from build123d import *

# Parameters (mm, degrees)
EXTRUDE_1_DEPTH      = 50
SKETCH_1_4_R         = 5.1
CUT_EXTRUDE_1_DEPTH  = 45
CUT_EXTRUDE_2_DEPTH  = 5
SKETCH_1_6_R         = 5.1
CUT_EXTRUDE_3_DEPTH  = 5
SKETCH_1_7_R         = 2.6
CUT_EXTRUDE_4_DEPTH  = 25
SKETCH_14_R          = 1.6
SKETCH_14_W          = 14
SKETCH_14_H          = 9
USB_DEPTH            = 5
SKETCH_16_W          = 24
SKETCH_16_H          = 24
CUT_EXTRUDE_12_DEPTH = 5
SKETCH_18_W          = 24
SKETCH_18_H          = 24
CUT_EXTRUDE_13_DEPTH = 5
EXTRUDE_2_DEPTH      = 40
EXTRUDE_3_DEPTH      = 2
SKETCH_29_4_R        = 2.85
SKETCH_29_4_R_2      = 1.15
EXTRUDE_4_DEPTH      = 5
SKETCH_29_5_R        = 3.4
SKETCH_29_5_R_2      = 1.2
EXTRUDE_5_DEPTH      = 6.5
CUT_EXTRUDE_START    = -2
SKETCH_29_6_R        = 1.15
SKETCH_29_6_R_2      = 1.2
CUT_EXTRUDE_14_DEPTH = 2


with BuildPart() as part:
    # Sketch 1 → Extrude 1 (new body)
    with BuildSketch(Plane.XY):
        with BuildLine():
            Line((-130, 82.5), (130, 82.5))
            ThreePointArc((130, 82.5), (145.909902577, 75.909902577), (152.5, 60))
            Line((152.5, 60), (152.5, -60))
            ThreePointArc((152.5, -60), (145.909902577, -75.909902577), (130, -82.5))
            Line((130, -82.5), (-130, -82.5))
            ThreePointArc((-130, -82.5), (-145.909902577, -75.909902577), (-152.5, -60))
            Line((-152.5, -60), (-152.5, 60))
            ThreePointArc((-152.5, 60), (-145.909902577, 75.909902577), (-130, 82.5))
        make_face()
    extrude(amount=EXTRUDE_1_DEPTH)

    # Sketch 1_4 → Cut-Extrude 1 (cut)
    with BuildSketch(Plane.XY):
        with BuildLine():
            Line((-130, 77.5), (130, 77.5))
            ThreePointArc((130, 77.5), (142.374368671, 72.374368671), (147.5, 60))
            Line((147.5, 60), (147.5, -60))
            ThreePointArc((147.5, -60), (142.374368671, -72.374368671), (130, -77.5))
            Line((130, -77.5), (-130, -77.5))
            ThreePointArc((-130, -77.5), (-142.374368671, -72.374368671), (-147.5, -60))
            Line((-147.5, -60), (-147.5, 60))
            ThreePointArc((-147.5, 60), (-142.374368671, 72.374368671), (-130, 77.5))
        make_face()
        with Locations(Location((130, 60, 0), (0, 0, 180))):
            Circle(SKETCH_1_4_R, mode=Mode.SUBTRACT)
        with Locations(Location((130, -60, 0), (0, 0, 180))):
            Circle(SKETCH_1_4_R, mode=Mode.SUBTRACT)
        with Locations(Location((-130, 60, 0), (0, 0, 180))):
            Circle(SKETCH_1_4_R, mode=Mode.SUBTRACT)
        with Locations(Location((-130, -60, 0), (0, 0, 180))):
            Circle(SKETCH_1_4_R, mode=Mode.SUBTRACT)
    extrude(amount=CUT_EXTRUDE_1_DEPTH, mode=Mode.SUBTRACT)

    # Sketch 1_5 → Cut-Extrude 2 (cut)
    with BuildSketch(Plane.XY):
        with BuildLine():
            ThreePointArc((-150.2, 60), (-144.28355698, 74.28355698), (-130, 80.2))
            Line((-130, 80.2), (130, 80.2))
            ThreePointArc((130, 80.2), (144.28355698, 74.28355698), (150.2, 60))
            Line((150.2, 60), (150.2, -60))
            ThreePointArc((150.2, -60), (144.28355698, -74.28355698), (130, -80.2))
            Line((130, -80.2), (-130, -80.2))
            ThreePointArc((-130, -80.2), (-144.28355698, -74.28355698), (-150.2, -60))
            Line((-150.2, -60), (-150.2, 60))
        make_face()
        with BuildLine():
            Line((-147.5, 60), (-147.5, -60))
            ThreePointArc((-147.5, -60), (-142.374368671, -72.374368671), (-130, -77.5))
            Line((-130, -77.5), (130, -77.5))
            ThreePointArc((130, -77.5), (142.374368671, -72.374368671), (147.5, -60))
            Line((147.5, -60), (147.5, 60))
            ThreePointArc((147.5, 60), (142.374368671, 72.374368671), (130, 77.5))
            Line((130, 77.5), (-130, 77.5))
            ThreePointArc((-130, 77.5), (-142.374368671, 72.374368671), (-147.5, 60))
        make_face(mode=Mode.SUBTRACT)
    extrude(amount=CUT_EXTRUDE_2_DEPTH, mode=Mode.SUBTRACT)

    # Sketch 1_6 → Cut-Extrude 3 (cut)
    with BuildSketch(Plane.XY):
        with Locations(Location((130, 60, 0), (0, 0, 180))):
            Circle(SKETCH_1_6_R)
        with Locations(Location((130, -60, 0), (0, 0, 180))):
            Circle(SKETCH_1_6_R)
        with Locations(Location((-130, 60, 0), (0, 0, 180))):
            Circle(SKETCH_1_6_R)
        with Locations(Location((-130, -60, 0), (0, 0, 180))):
            Circle(SKETCH_1_6_R)
    extrude(amount=CUT_EXTRUDE_3_DEPTH, mode=Mode.SUBTRACT)

    # Sketch 1_7 → Cut-Extrude 4 (cut)
    with BuildSketch(Plane.XY):
        with Locations((-130, -60)):
            Circle(SKETCH_1_7_R)
        with Locations((130, 60)):
            Circle(SKETCH_1_7_R)
        with Locations((130, -60)):
            Circle(SKETCH_1_7_R)
        with Locations((-130, 60)):
            Circle(SKETCH_1_7_R)
    extrude(amount=CUT_EXTRUDE_4_DEPTH, mode=Mode.SUBTRACT)

    # Sketch 14 → USB (cut)
    with BuildSketch(Plane.XZ.offset(82.5)):
        with Locations(Location((-70.9, 38, 0), (0, 0, 270))):
            Circle(SKETCH_14_R)
        with Locations(Location((-89.1, 38, 0), (0, 0, 270))):
            Circle(SKETCH_14_R)
        with Locations((-80, 38)):
            Rectangle(SKETCH_14_W, SKETCH_14_H)
    extrude(amount=-USB_DEPTH, mode=Mode.SUBTRACT)

    # Sketch 16 → Cut-Extrude 12 (cut)
    with BuildSketch(Plane(origin=(152.5, 0, 0), x_dir=(0, 0, -1), z_dir=(1, 0, 0))):
        with Locations((-30, -38)):
            Rectangle(SKETCH_16_W, SKETCH_16_H)
    extrude(amount=-CUT_EXTRUDE_12_DEPTH, mode=Mode.SUBTRACT)

    # Sketch 18 → Cut-Extrude 13 (cut)
    with BuildSketch(Plane.ZY.offset(152.5)):
        with Locations((30, -38)):
            Rectangle(SKETCH_18_W, SKETCH_18_H)
    extrude(amount=-CUT_EXTRUDE_13_DEPTH, mode=Mode.SUBTRACT)

    # Sketch 19 → Extrude 2 (add)
    with BuildSketch(Plane(origin=(0, 0, 45), x_dir=(-1, 0, 0), z_dir=(0, 0, -1))):
        with BuildLine():
            Line((-103, 40), (-18, 40))
            ThreePointArc((-18, 40), (-14, 36), (-18, 32))
            Line((-18, 32), (-103, 32))
            ThreePointArc((-103, 32), (-107, 36), (-103, 40))
        make_face()
        with BuildLine():
            Line((103, 40), (18, 40))
            ThreePointArc((18, 40), (14, 36), (18, 32))
            Line((18, 32), (103, 32))
            ThreePointArc((103, 32), (107, 36), (103, 40))
        make_face()
        with BuildLine():
            Line((-103, -20), (-23, -20))
            ThreePointArc((-23, -20), (-19, -24), (-23, -28))
            Line((-23, -28), (-103, -28))
            ThreePointArc((-103, -28), (-107, -24), (-103, -20))
        make_face()
        with BuildLine():
            Line((103, -20), (23, -20))
            ThreePointArc((23, -20), (19, -24), (23, -28))
            Line((23, -28), (103, -28))
            ThreePointArc((103, -28), (107, -24), (103, -20))
        make_face()
    extrude(amount=EXTRUDE_2_DEPTH)

    # Sketch 29 → Extrude 3 (add)
    with BuildSketch(Plane(origin=(0, 0, 45), x_dir=(-1, 0, 0), z_dir=(0, 0, -1))):
        Polygon((-14.35, -45.2), (14.35, -45.2), (14.35, -18.5), (12.85, -18.5), (12.85, -20), (12.85, -43.7), (-12.85, -43.7), (-12.85, -20), (-12.85, -18.5), (-14.35, -18.5), align=None)
    extrude(amount=EXTRUDE_3_DEPTH)

    # Sketch 29_4 → Extrude 4 (add)
    # profile 1 of 2: a face of its own
    with BuildSketch(Plane(origin=(0, 0, 45), x_dir=(-1, 0, 0), z_dir=(0, 0, -1))):
        with Locations(Location((-17.5, -31.85, 0), (0, 0, 180))):
            Circle(SKETCH_29_4_R)
        with Locations((-17.5, -31.85)):
            Circle(SKETCH_29_4_R_2, mode=Mode.SUBTRACT)
    # profile 2 of 2: a face of its own
    with BuildSketch(Plane(origin=(0, 0, 45), x_dir=(-1, 0, 0), z_dir=(0, 0, -1))):
        with Locations((17.5, -31.85)):
            Circle(SKETCH_29_4_R)
        with Locations(Location((17.5, -31.85, 0), (0, 0, 180))):
            Circle(SKETCH_29_4_R_2, mode=Mode.SUBTRACT)
    extrude(amount=EXTRUDE_4_DEPTH)

    # Sketch 29_5 → Extrude 5 (add)
    # profile 1 of 4: a face of its own
    with BuildSketch(Plane(origin=(0, 0, 45), x_dir=(-1, 0, 0), z_dir=(0, 0, -1))):
        with Locations(Location((-30, 20, 0), (0, 0, 180))):
            Circle(SKETCH_29_5_R)
        with Locations(Location((-30, 20, 0), (0, 0, 180))):
            Circle(SKETCH_29_5_R_2, mode=Mode.SUBTRACT)
    # profile 2 of 4: a face of its own
    with BuildSketch(Plane(origin=(0, 0, 45), x_dir=(-1, 0, 0), z_dir=(0, 0, -1))):
        with Locations(Location((-30, -10, 0), (0, 0, 180))):
            Circle(SKETCH_29_5_R)
        with Locations(Location((-30, -10, 0), (0, 0, 180))):
            Circle(SKETCH_29_5_R_2, mode=Mode.SUBTRACT)
    # profile 3 of 4: a face of its own
    with BuildSketch(Plane(origin=(0, 0, 45), x_dir=(-1, 0, 0), z_dir=(0, 0, -1))):
        with Locations(Location((30, 20, 0), (0, 0, 180))):
            Circle(SKETCH_29_5_R)
        with Locations(Location((30, 20, 0), (0, 0, 180))):
            Circle(SKETCH_29_5_R_2, mode=Mode.SUBTRACT)
    # profile 4 of 4: a face of its own
    with BuildSketch(Plane(origin=(0, 0, 45), x_dir=(-1, 0, 0), z_dir=(0, 0, -1))):
        with Locations(Location((30, -10, 0), (0, 0, 180))):
            Circle(SKETCH_29_5_R)
        with Locations(Location((30, -10, 0), (0, 0, 180))):
            Circle(SKETCH_29_5_R_2, mode=Mode.SUBTRACT)
    extrude(amount=EXTRUDE_5_DEPTH)

    # Sketch 29_6 → Cut-Extrude 14 (cut)
    with BuildSketch(Plane(origin=(0, 0, 45), x_dir=(-1, 0, 0), z_dir=(0, 0, -1)).offset(CUT_EXTRUDE_START)):
        with Locations((17.5, -31.85)):
            Circle(SKETCH_29_6_R)
        with Locations((-17.5, -31.85)):
            Circle(SKETCH_29_6_R)
        with Locations(Location((30, -10, 0), (0, 0, 180))):
            Circle(SKETCH_29_6_R_2)
        with Locations(Location((-30, -10, 0), (0, 0, 180))):
            Circle(SKETCH_29_6_R_2)
        with Locations(Location((-30, 20, 0), (0, 0, 180))):
            Circle(SKETCH_29_6_R_2)
        with Locations(Location((30, 20, 0), (0, 0, 180))):
            Circle(SKETCH_29_6_R_2)
    extrude(amount=CUT_EXTRUDE_14_DEPTH, mode=Mode.SUBTRACT)


solid = part.part
The listing builds one solid part. Answer for the finished solid, in the listing's coordinates (mm). Coordinates: 2 decimals unless noted, no trailing zeros. Loops run counter-clockwise (first coordinate to the right, second up) from the corner with the lowest first, then second, coordinate; pieces in that order, holes last. Notation, with made-up numbers: (82, 56.5) -> (136, 56.5) arc R24 ccw to (136, 76.5) -> close; hole circle Ø8 at (75.25, 13.25). An arc over 180 degrees is marked (long way). Write item = value, one per line. Start each with the question number.
1) Given pin 1 Ø10 at (x, y) = (121.5, -23.5) entering from -Z; pin 2 Ø4 at (x, y) = (-129, 60) entering from -Z; pin 3 Ø1.9 at (x, y) = (30, 19.5) entering from -Z, each flat-ended and moving along its own axis, determine where each tip first touches the part or whether it passes through.
2) Straight lines are drawn through the part: line 1 (X direction, y = 60, z = 11.75); line 2 (X direction, y = -10, z = 41.5); line 3 (Y direction, x = -72.5, z = 33). For each, find the intervals that lie inside material, in ascending order. Write a range as from..to.
3) A cutting plane is placed at B-B (x = -54.5). Give the vertices of the cut face in (y, z), then the cut area to 3 significant figures.
4) A cutting plane is placed at A-A (y = 48). Give the vertices of the cut face in (x, z).
5) The mould has two halves that part along Y. Classify faces 1 (the face through (2, 1, 50)), 2 (the face through (-28.5, 20, 38.5)), 3 (the face through (2, -82.5, 25)): released by +Y, released by -Y, zero draft, split by the parting line, or undercut.
Responses:
q1.pin_1 = 45
q1.pin_2 = 5
q1.pin_3 = 38.5
q2.line_1 = -152.5..-147.5, -135.1..-132.6, -127.4..-124.9, 124.9..127.4, 132.6..135.1, 147.5..152.5
q2.line_2 = -152.5..-147.5, -33.4..-31.2, -28.8..-26.6, 26.6..28.8, 31.2..33.4, 147.5..152.5
q2.line_3 = -82.5..-77.5, -28..-20, 32..40, 77.5..82.5
q3.outline = (-82.5, 0) -> (-80.2, 0) -> (-80.2, 5) -> (-77.5, 5) -> (-77.5, 45) -> (-28, 45) -> (-28, 5) -> (-20, 5) -> (-20, 45) -> (32, 45) -> (32, 5) -> (40, 5) -> (40, 45) -> (77.5, 45) -> (77.5, 5) -> (80.2, 5) -> (80.2, 0) -> (82.5, 0) -> (82.5, 50) -> (-82.5, 50) -> close
q3.area = 1,890 mm²
q4.outline = (-152.5, 0) -> (-150.2, 0) -> (-150.2, 5) -> (-147.5, 5) -> (-147.5, 45) -> (147.5, 45) -> (147.5, 5) -> (150.2, 5) -> (150.2, 0) -> (152.5, 0) -> (152.5, 50) -> (-152.5, 50) -> close
q5.face_1 = zero draft
q5.face_2 = undercut
q5.face_3 = released by -Y
